from build123d import *

# Parameters (mm, degrees)
BOSS_EXTRUDE1_DEPTH     = 5
SKETCH2_R               = 1.75
CUT_EXTRUDE1_DEPTH      = 5
SKETCH3_R               = 1.75
CUT_EXTRUDE2_DEPTH      = 159.823801743
FILL_PATTERN1_OUTLINE_R = 1.75
FILL_PATTERN1_DEPTH     = 5


# Read off the part's stored shape, not the designer's step: Fill Pattern1
with BuildPart() as part:
    # Sketch1 → Boss-Extrude1 (new body)
    with BuildSketch(Plane.XY):
        Polygon((103.923048454, -60), (103.923048454, 60), (0, 120), (-103.923048454, 60), (-103.923048454, -60), (0, -120), align=None)
    extrude(amount=BOSS_EXTRUDE1_DEPTH)

    # Sketch2 → Cut-Extrude1 (cut)
    with BuildSketch(Plane.XY.offset(5)):
        with Locations((-99.592921435, 57.5)):
            Circle(SKETCH2_R)
        with Locations((-95.262794416, 55)):
            Circle(SKETCH2_R)
        with Locations(Location((95.262794416, 55, 0), (0, 0, 180))):
            Circle(SKETCH2_R)
        with Locations(Location((99.592921435, 57.5, 0), (0, 0, 180))):
            Circle(SKETCH2_R)
        with Locations((99.592921435, -57.5)):
            Circle(SKETCH2_R)
        with Locations((95.262794416, -55)):
            Circle(SKETCH2_R)
        with Locations(Location((-95.262794416, -55, 0), (0, 0, 180))):
            Circle(SKETCH2_R)
        with Locations(Location((-99.592921435, -57.5, 0), (0, 0, 180))):
            Circle(SKETCH2_R)
        with Locations((0, -115)):
            Circle(SKETCH2_R)
        with Locations((0, -110)):
            Circle(SKETCH2_R)
        with Locations(Location((0, 115, 0), (0, 0, 180))):
            Circle(SKETCH2_R)
        with Locations(Location((0, 110, 0), (0, 0, 180))):
            Circle(SKETCH2_R)
    extrude(amount=-CUT_EXTRUDE1_DEPTH, mode=Mode.SUBTRACT)

    # Sketch3 → Cut-Extrude2 (cut, through all)
    with BuildSketch(Plane.XY.offset(5)):
        Circle(SKETCH3_R)
    extrude(amount=-CUT_EXTRUDE2_DEPTH, mode=Mode.SUBTRACT)

    # Fill Pattern1 outline → Fill Pattern1 (cut)
    with BuildSketch(Plane.XY):
        with Locations((-27.49545417, -15.874507866)):
            Circle(FILL_PATTERN1_OUTLINE_R)
        with Locations((-54.990908339, -31.749015733)):
            Circle(FILL_PATTERN1_OUTLINE_R)
        with Locations((-82.486362509, -47.623523599)):
            Circle(FILL_PATTERN1_OUTLINE_R)
        with Locations((70.865416206, 4.253561563)):
            Circle(FILL_PATTERN1_OUTLINE_R)
        with Locations((-70.865416206, -4.253561563)):
            Circle(FILL_PATTERN1_OUTLINE_R)
        with Locations((82.486362509, 47.623523599)):
            Circle(FILL_PATTERN1_OUTLINE_R)
        with Locations((54.990908339, 31.749015733)):
            Circle(FILL_PATTERN1_OUTLINE_R)
        with Locations((27.49545417, 15.874507866)):
            Circle(FILL_PATTERN1_OUTLINE_R)
        with Locations((4.253561563, -70.865416206)):
            Circle(FILL_PATTERN1_OUTLINE_R)
        with Locations((31.749015733, -54.990908339)):
            Circle(FILL_PATTERN1_OUTLINE_R)
        with Locations((59.244469903, -39.116400473)):
            Circle(FILL_PATTERN1_OUTLINE_R)
        with Locations((86.739924072, -23.241892607)):
            Circle(FILL_PATTERN1_OUTLINE_R)
        with Locations((-39.116400473, -59.244469903)):
            Circle(FILL_PATTERN1_OUTLINE_R)
        with Locations((-11.620946303, -43.369962036)):
            Circle(FILL_PATTERN1_OUTLINE_R)
        with Locations((15.874507866, -27.49545417)):
            Circle(FILL_PATTERN1_OUTLINE_R)
        with Locations((43.369962036, -11.620946303)):
            Circle(FILL_PATTERN1_OUTLINE_R)
        with Locations((-4.253561563, 70.865416206)):
            Circle(FILL_PATTERN1_OUTLINE_R)
        with Locations((-31.749015733, 54.990908339)):
            Circle(FILL_PATTERN1_OUTLINE_R)
        with Locations((-59.244469903, 39.116400473)):
            Circle(FILL_PATTERN1_OUTLINE_R)
        with Locations((-86.739924072, 23.241892607)):
            Circle(FILL_PATTERN1_OUTLINE_R)
        with Locations((39.116400473, 59.244469903)):
            Circle(FILL_PATTERN1_OUTLINE_R)
        with Locations((11.620946303, 43.369962036)):
            Circle(FILL_PATTERN1_OUTLINE_R)
        with Locations((-15.874507866, 27.49545417)):
            Circle(FILL_PATTERN1_OUTLINE_R)
        with Locations((-43.369962036, 11.620946303)):
            Circle(FILL_PATTERN1_OUTLINE_R)
        with Locations((23.241892607, 86.739924072)):
            Circle(FILL_PATTERN1_OUTLINE_R)
        with Locations((-23.241892607, -86.739924072)):
            Circle(FILL_PATTERN1_OUTLINE_R)
    extrude(amount=FILL_PATTERN1_DEPTH, mode=Mode.SUBTRACT)


solid = part.part
Could you check a few things on this model? Use its own coordinates, in mm. Give positions to 0.01 mm unless a question says otherwise; leave off trailing zeros.
1. Suppose I cut it at A-A (z = 2). State how many separate pieces and enclosed holes the cut face has, plus the area to 3 significant figures.
Answers below:
separate pieces: 1
enclosed holes: 39
area: 37,000 mm2
2. I need wall thicknesses on L1, parallel to X at y = 48, z = 4.5; L2, parallel to X at y = -43, z = 3.65; L3, parallel to Y at x = 1, z = 4.55. Which ranges of each line are inside material? Lowest first, please.
Answers below:
L1: x = -103.92 to 80.78, 84.2 to 103.92
L2: x = -103.92 to -13.33, -9.91 to 103.92
L3: y = -119.42 to -116.44, -113.56 to -111.44, -108.56 to -1.44, 1.44 to 108.56, 111.44 to 113.56, 116.44 to 119.42
3. For pin 1 (3 mm diameter, centred on x = 11.62, y = 43.37, fed in from -Z); pin 2 (3 mm diameter, centred on x = 78, z = 3.5, fed in from -Y); pin 3 (2 mm diameter, centred on x = -4, z = 1, fed in from +Y), each with a flat end and sliding along its axis, tell me the tip position at first contact or that it passes through.
Answers below:
pin 1: passes through
pin 2: stops at y = -75.83
pin 3: stops at y = 118.27
4. Thinking about a two-plate mould opening in Z: for faces 1 (the flat face through (-1, 2, 0)), 2 (the flat face through (-51.234, 90.42, 2.465)), 3 (the flat face through (-1, 2, 5)), which applies, +Z half, -Z half, draft (parallel to the pull), parting line (faces both ways), or undercut?
Answers below:
face 1: -Z half
face 2: draft
face 3: +Z half
